from build123d import *

# Parameters (mm, degrees)
F1_DEPTH = 60
F2_SIZE2 = 46.1504797148
F2_SIZE  = 55
F3_DEPTH = 30
F5_DEPTH = 85


with BuildPart() as f1:
    # F0 (on Top) → F1 (new body)
    with BuildSketch(Plane.XY):
        with BuildLine():
            Line((-50, -40), (50, -40))
            Line((50, -40), (50, 20))
            ThreePointArc((50, 20), (44.1421356237, 34.1421356237), (30, 40))
            Line((30, 40), (-30, 40))
            ThreePointArc((-30, 40), (-44.1421356237, 34.1421356237), (-50, 20))
            Line((-50, 20), (-50, -40))
        make_face()
    extrude(amount=F1_DEPTH)

    # F2
    f2_edges = [f1.edges().sort_by_distance(p)[0] for p in [
        (0, -40, 60),
    ]]
    f2_side = f1.faces().sort_by_distance((0, -40, 30))[0]
    chamfer(f2_edges, length=F2_SIZE, length2=F2_SIZE2, reference=f2_side)

    # F3 (add): a face of the model
    f3_faces = [f1.faces().sort_by_distance(p)[0] for p in [
        (0, 22.4096547689, 60),
    ]]
    extrude(f3_faces, amount=F3_DEPTH)

    # F4 (on face) → F5 (cut)
    with BuildSketch(Plane.XY.offset(90)):
        with BuildLine():
            Line((30, 36), (2, 36))
            Line((2, 36), (2, 10.1504797148))
            Line((2, 10.1504797148), (46, 10.1504797148))
            Line((46, 10.1504797148), (46, 20))
            ThreePointArc((46, 20), (41.313708499, 31.313708499), (30, 36))
        make_face()
        with BuildLine():
            Line((-2, 36), (-30, 36))
            ThreePointArc((-30, 36), (-41.313708499, 31.313708499), (-46, 20))
            Line((-46, 20), (-46, 10.1504797148))
            Line((-46, 10.1504797148), (-2, 10.1504797148))
            Line((-2, 10.1504797148), (-2, 36))
        make_face()
    extrude(amount=-F5_DEPTH, mode=Mode.SUBTRACT)


solid = f1.part
Work out the finished part from the listing and answer in its coordinate system (mm). A direction names the side the tool comes from. Round coordinates to 2 decimals unless told otherwise and drop trailing zeros. Loops run counter-clockwise (first coordinate to the right, second up) from the corner with the lowest first, then second, coordinate; pieces in that order, holes last. Notation, with made-up numbers: (3, 89) - (35, 89) arc R23 ccw to (35, 97) - close; hole circle Ø4 at (35.25, 29.5). An arc over 180 degrees is marked (long way). Use one line per item in the form item = value. Start each with the question number.
(1) Which of the six approach directions +Z, -Z, +X, -X, +Y, -Y give full straight-line access (tool end or side, diameter ignored) to faces 1 (the face through (41.437, 31.189, 48.095)), 2 (the face through (-1, 6.15, 75)), 3 (the face through (-50, -3, 34))?
(2) Flat-ended cylindrical pins translate along their axes: P1, Ø5, axis at x = 12.5, y = 20.5, coming from the +Z side; P2, Ø8.5, axis at x = -11.5, z = 38.5, coming from the -Y side; P3, Ø24, axis at x = -20, z = 68, coming from the -Y side; P4, Ø12, axis at x = 34, z = 24.5, coming from the +Y side. Find the tip coordinate at first contact, or state that the pin passes through.
(3) Determine the mould class of faces 4 (the face through (46, 15, 48)), 5 (the face through (44.297, 33.986, 44.37)), 6 (the face through (0, 40, 44)) for opening direction X: +X half, -X half, draft (parallel to the pull), parting line (faces both ways), or undercut.
(4) Consider line 1 (X direction, y = 21, z = 24); line 2 (Y direction, x = 10.5, z = 69.5); line 3 (X direction, y = 30.5, z = 68). Determine where each line is inside the solid, lowest interval first.
(5) Find section A-A on z = 73. Determine the outline of the cut face in (x, y), and give its area (3 significant figures).
(6) Find section D-D on z = 46. Determine the outline of the cut face in (x, y).
(7) Find section B-B on x = 16.5. Determine the outline of the cut face in (y, z), and give its area (3 significant figures).
(8) Find section C-C on y = 13.5. Determine the outline of the cut face in (x, z), and give its area (3 significant figures).
Answer list:
q1.face_1 = +Z
q1.face_2 = +Z, +X, -X, -Y
q1.face_3 = +Z, -Z, -X, +Y, -Y
q2.P1 = 5
q2.P2 = -15.46
q2.P3 = 2.79
q2.P4 = 40
q3.face_4 = undercut
q3.face_5 = +X half
q3.face_6 = draft
q4.line_1 = -49.97 to -45.97, -2 to 2, 45.97 to 49.97
q4.line_2 = 6.15 to 10.15, 36 to 40
q4.line_3 = -47.02 to -42.07, -2 to 2, 42.07 to 47.02
q5.outline = (-50, 6.15) - (50, 6.15) - (50, 20) arc R20 ccw to (30, 40) - (-30, 40) arc R20 ccw to (-50, 20) - close; hole (-46, 10.15) - (-2, 10.15) - (-2, 36) - (-30, 36) arc R16 ccw to (-46, 20) - close; hole (2, 10.15) - (46, 10.15) - (46, 20) arc R16 ccw to (30, 36) - (2, 36) - close
q5.area = 1,050 mm^2
q6.outline = (-50, -5.6) - (50, -5.6) - (50, 20) arc R20 ccw to (30, 40) - (-30, 40) arc R20 ccw to (-50, 20) - close; hole (-46, 10.15) - (-2, 10.15) - (-2, 36) - (-30, 36) arc R16 ccw to (-46, 20) - close; hole (2, 10.15) - (46, 10.15) - (46, 20) arc R16 ccw to (30, 36) - (2, 36) - close
q7.outline = (-40, 0) - (40, 0) - (40, 90) - (36, 90) - (36, 5) - (10.15, 5) - (10.15, 90) - (6.15, 90) - (6.15, 60) - (-40, 5) - close
q7.area = 2,350 mm^2
q8.outline = (-50, 0) - (50, 0) - (50, 90) - (46, 90) - (46, 5) - (2, 5) - (2, 90) - (-2, 90) - (-2, 5) - (-46, 5) - (-46, 90) - (-50, 90) - close
q8.area = 1,520 mm^2
